Check sheet for the modelled part. Datum: model origin and axes. Units: mm. A direction names the side the tool comes from. Round coordinates to 2 decimals unless told otherwise and drop trailing zeros. Order: outer loops, then holes, each group sorted by start corner. A loop starts at its lowest first (then second) coordinate and runs counter-clockwise, first axis right, second up. Notation, with made-up numbers: M -17,41.25 L -2,41.25 A13 ccw -2,50.25 Z; hole C -36.5,-9.5 d7. An arc over 180 degrees is marked long. One line per item, written item: value. Start each with the question number.
(1) Cross-section at B-B, the plane y = 31. Enter the section's corners in (x, z), and give its area (3 significant figures).
(2) Cross-section at D-D, the plane z = 0. Enter the section's corners in (x, y).
(3) Cross-section at A-A, the plane z = 3.5. Enter the section's corners in (x, y).
(4) Access from +Z, -Z, +X, -X, +Y, -Y to the whole of each face (thin tool, end or side, straight path). Record for faces 5 (the face through (-8.4, 5.03, 7.11)), 6 (the face through (0, 0, 7)), 7 (the face through (15, 21.5, -8)), 8 (the face through (-0.225, 12.782, -9.635)), 9 (the face through (0, 21.5, 7)).
(5) Thickness scan on L1, parallel to X at y = 1.8, z = 0; L2, parallel to Z at x = -13.5, y = 1.8; L3, parallel to Z at x = -12, y = 6. Record the ranges inside material, lowest first.
(6) Depth check by flat-ended pin: pin 1 Ø1 at (x, z) = (2.5, 6.5) entering from +Y; pin 2 Ø5 at (y, z) = (9.5, 2) entering from +X; pin 3 Ø1.6 at (x, z) = (-2, -7) entering from +Y; pin 4 Ø0.7 at (x, y) = (-9, 22) entering from +Z. Enter the tip coordinate at first touch or a pass-through.
(7) Cross-section at C-C, the plane x = -13.5. Enter the section's corners in (y, z), and give its area (3 significant figures).
(8) Release check for a two-part mould opening along X. For faces 1 (the face through (-9.1, 21.4, -9.1)), 2 (the face through (-4.91, 7.606, -7.249)), 3 (the face through (-6.593, 22.291, -8.128)), 4 (the face through (-0.1, 10, -9.1)) record: released by +X, released by -X, zero draft, split by the parting line, or undercut.
from build123d import *

# Parameters (mm, degrees)
CROQUIS1_W                        = 5
CROQUIS1_H                        = 16.2
SALIENTE_EXTRUIR1_DEPTH           = 3
SALIENTE_EXTRUIR1_2_DEPTH         = 3
CROQUIS2_R                        = 0.8
CORTAR_EXTRUIR2_DEPTH             = 3
CROQUIS4_W                        = 32.2
CROQUIS4_H                        = 2
SALIENTE_EXTRUIR2_DEPTH           = 18.5
SALIENTE_EXTRUIR2_DEPTH_BACK      = 3
CROQUIS5_W                        = 5
CROQUIS5_H                        = 12.2
SALIENTE_EXTRUIR3_DEPTH           = 2
SALIENTE_EXTRUIR4_DEPTH           = 32.2
CORTAR_EXTRUIR3_REACH             = 35.7
CROQUIS8_W                        = 22.2
CROQUIS8_H                        = 2
CORTAR_EXTRUIR3_DIRECTION_2_DEPTH = 1
CORTAR_EXTRUIR4_REACH             = 20.2
CROQUIS9_R                        = 0.8
CROQUIS10_R                       = 0.8
SALIENTE_EXTRUIR5_DEPTH           = 2
SALIENTE_EXTRUIR7_DEPTH           = 32.2
CORTAR_EXTRUIR5_DEPTH             = 19.2
CORTAR_EXTRUIR9_DEPTH             = 0.3
CORTAR_EXTRUIR9_DIRECTION_2_REACH = 14.2
CROQUIS21_W                       = 32.2
CROQUIS21_H                       = 12.2
CORTAR_EXTRUIR10_DEPTH            = 0.4


with BuildPart() as part:
    # Croquis1 → Saliente-Extruir1 (new body)
    with BuildSketch(Plane(origin=(0, 0, 0), x_dir=(1, 0, 0), z_dir=(0, 1, 0))):
        with Locations((-13.6, 0)):
            Rectangle(CROQUIS1_W, CROQUIS1_H)
    extrude(amount=SALIENTE_EXTRUIR1_DEPTH)


with BuildPart() as body_2:
    # Croquis1 → Saliente-Extruir1 2 (new body)
    with BuildSketch(Plane(origin=(0, 0, 0), x_dir=(1, 0, 0), z_dir=(0, 1, 0))):
        with Locations((13.6, 0)):
            Rectangle(CROQUIS1_W, CROQUIS1_H)
    extrude(amount=SALIENTE_EXTRUIR1_2_DEPTH)


with BuildPart() as cortar_extruir2_tool:
    # Croquis2 → Cortar-Extruir2 (new body)
    with BuildSketch(Plane(origin=(0, 3, 0), x_dir=(1, 0, 0), z_dir=(0, 1, 0))):
        with Locations((-13.5, 0)):
            Circle(CROQUIS2_R)
        with Locations((14, 0)):
            Circle(CROQUIS2_R)
    extrude(amount=-CORTAR_EXTRUIR2_DEPTH)


with BuildPart() as part_1:
    add(part.part)

    # Cortar-Extruir2: cut by cortar_extruir2_tool
    add(cortar_extruir2_tool.part, mode=Mode.SUBTRACT)



with BuildPart() as body_2_1:
    add(body_2.part)

    # Cortar-Extruir2: cut by cortar_extruir2_tool
    add(cortar_extruir2_tool.part, mode=Mode.SUBTRACT)


with BuildPart() as part_2:
    add(part_1.part)

    add(body_2_1.part)  # Saliente-Extruir2 merges body 2
    # Croquis4 → Saliente-Extruir2 (add, two sides)
    with BuildSketch(Plane(origin=(0, 3, 0), x_dir=(1, 0, 0), z_dir=(0, 1, 0))) as saliente_extruir2_sk:
        with Locations((0, 7.1)):
            Rectangle(CROQUIS4_W, CROQUIS4_H)
        with Locations((0, -7.1)):
            Rectangle(CROQUIS4_W, CROQUIS4_H)
    extrude(amount=SALIENTE_EXTRUIR2_DEPTH)
    extrude(saliente_extruir2_sk.sketch, amount=-SALIENTE_EXTRUIR2_DEPTH_BACK)

    # Croquis5 → Saliente-Extruir3 (add)
    with BuildSketch(Plane.XY.offset(8.1)):
        with Locations((13.6, 27.6)):
            Rectangle(CROQUIS5_W, CROQUIS5_H)
        with Locations((-13.6, 27.6)):
            Rectangle(CROQUIS5_W, CROQUIS5_H)
    extrude(amount=-SALIENTE_EXTRUIR3_DEPTH)

    # Croquis7 → Saliente-Extruir4 (add, through all)
    with BuildSketch(Plane.ZY.offset(16.1)):
        with BuildLine():
            Line((10.1, 33.7), (8.1, 33.7))
            Line((8.1, 33.7), (8.1, 7.353005636))
            ThreePointArc((8.1, 7.353005636), (8.248733131, 9.983124325), (8.693036056, 12.579706844))
            Line((8.693036056, 12.579706844), (9.506963944, 16.120293156))
            ThreePointArc((9.506963944, 16.120293156), (9.951266869, 18.716875675), (10.1, 21.346994364))
            Line((10.1, 21.346994364), (10.1, 33.7))
        make_face()
    extrude(amount=-SALIENTE_EXTRUIR4_DEPTH)

    # Croquis8 → Cortar-Extruir3 (cut, up to next)
    with BuildSketch(Plane(origin=(0, 33.7, 0), x_dir=(1, 0, 0), z_dir=(0, 1, 0)), mode=Mode.PRIVATE) as cortar_extruir3_sk1:
        with Locations((0, -9.1)):
            Rectangle(CROQUIS8_W, CROQUIS8_H)
    cortar_extruir3_tool1 = extrude(cortar_extruir3_sk1.sketch, amount=-CORTAR_EXTRUIR3_REACH, mode=Mode.PRIVATE) & part_2.part
    add(cortar_extruir3_tool1.solids().sort_by_distance((0, 33.7, 9.1))[0], mode=Mode.SUBTRACT)

    # Croquis8 → Cortar-Extruir3 direction 2 (cut)
    with BuildSketch(Plane(origin=(0, 33.7, 0), x_dir=(1, 0, 0), z_dir=(0, 1, 0))):
        with Locations((0, -9.1)):
            Rectangle(CROQUIS8_W, CROQUIS8_H)
    extrude(amount=CORTAR_EXTRUIR3_DIRECTION_2_DEPTH, mode=Mode.SUBTRACT)

    # Croquis9 → Cortar-Extruir4 (cut, up to next)
    with BuildSketch(Plane.XY.offset(10.1), mode=Mode.PRIVATE) as cortar_extruir4_sk1:
        with Locations((-13.85, 27.95)):
            Circle(CROQUIS9_R)
    cortar_extruir4_tool1 = extrude(cortar_extruir4_sk1.sketch, amount=-CORTAR_EXTRUIR4_REACH, mode=Mode.PRIVATE) & part_2.part
    add(cortar_extruir4_tool1.solids().sort_by_distance((-13.85, 27.95, 10.1))[0], mode=Mode.SUBTRACT)
    # Croquis9 → Cortar-Extruir4 (cut, up to next)
    with BuildSketch(Plane.XY.offset(10.1), mode=Mode.PRIVATE) as cortar_extruir4_sk2:
        with Locations((13.85, 27.95)):
            Circle(CROQUIS9_R)
    cortar_extruir4_tool2 = extrude(cortar_extruir4_sk2.sketch, amount=-CORTAR_EXTRUIR4_REACH, mode=Mode.PRIVATE) & part_2.part
    add(cortar_extruir4_tool2.solids().sort_by_distance((13.85, 27.95, 10.1))[0], mode=Mode.SUBTRACT)

    # Croquis10 → Saliente-Extruir5 (add, symmetric)
    with BuildSketch(Plane(origin=(0, 0, -8.1), x_dir=(-1, 0, 0), z_dir=(0, 0, -1))):
        with BuildLine():
            Line((-10.633991508, 23.582443769), (-7.130262645, 28.458778116))
            ThreePointArc((-7.130262645, 28.458778116), (-5.478846803, 29.471128305), (-3.6, 29))
            Line((-3.6, 29), (2.4, 24.5))
            ThreePointArc((2.4, 24.5), (6.65658351, 22.269750529), (11.4, 21.5))
            Line((11.4, 21.5), (-14.694516799, 21.5))
            ThreePointArc((-14.694516799, 21.5), (-12.412826763, 22.050967456), (-10.633991508, 23.582443769))
        make_face()
        with Locations((-5.1, 27)):
            Circle(CROQUIS10_R, mode=Mode.SUBTRACT)
    extrude(amount=SALIENTE_EXTRUIR5_DEPTH, both=True)

    # Croquis13 → Saliente-Extruir7 (add, through all)
    with BuildSketch(Plane.ZY.offset(16.1)):
        with BuildLine():
            Line((-8.1, 21.5), (-10.1, 21.5))
            Line((-10.1, 21.5), (-10.1, 18.465682976))
            ThreePointArc((-10.1, 18.465682976), (-9.929666433, 15.016866347), (-9.420323649, 11.601618246))
            Line((-9.420323649, 11.601618246), (-8.779676351, 8.398381754))
            ThreePointArc((-8.779676351, 8.398381754), (-8.270333567, 4.983133653), (-8.1, 1.534317024))
            Line((-8.1, 1.534317024), (-8.1, 21.5))
        make_face()
    extrude(amount=-SALIENTE_EXTRUIR7_DEPTH)

    # Croquis14 → Cortar-Extruir5 (cut, through all)
    with BuildSketch(Plane.XY.offset(8.1)):
        with BuildLine():
            Line((-9, 15.116941663), (-9, 5.945455337))
            ThreePointArc((-9, 5.945455337), (-8.38417979, 5.022197037), (-7.295188221, 5.236060978))
            Line((-7.295188221, 5.236060978), (-2.457737974, 10.042262026))
            ThreePointArc((-2.457737974, 10.042262026), (-2.499999997, 10.499882305), (-2.457781062, 10.95750656))
            Line((-2.457781062, 10.95750656), (-7.290605641, 15.821753441))
            ThreePointArc((-7.290605641, 15.821753441), (-8.381186071, 16.041440002), (-9, 15.116941663))
        make_face()
        with BuildLine():
            Line((-5.263939022, 17.795188221), (-0.457737974, 12.957737974))
            ThreePointArc((-0.457737974, 12.957737974), (-0.000117695, 12.999999997), (0.45750656, 12.957781062))
            Line((0.45750656, 12.957781062), (5.321753441, 17.790605641))
            ThreePointArc((5.321753441, 17.790605641), (5.541440002, 18.881186071), (4.616941663, 19.5))
            Line((4.616941663, 19.5), (-4.554544663, 19.5))
            ThreePointArc((-4.554544663, 19.5), (-5.477802963, 18.88417979), (-5.263939022, 17.795188221))
        make_face()
        with BuildLine():
            Line((7.295188221, 15.763939022), (2.457737974, 10.957737974))
            ThreePointArc((2.457737974, 10.957737974), (2.499999997, 10.500117695), (2.457781062, 10.04249344))
            Line((2.457781062, 10.04249344), (7.290605641, 5.178246559))
            ThreePointArc((7.290605641, 5.178246559), (8.381186071, 4.958559998), (9, 5.883058337))
            Line((9, 5.883058337), (9, 15.054544663))
            ThreePointArc((9, 15.054544663), (8.38417979, 15.977802963), (7.295188221, 15.763939022))
        make_face()
        with BuildLine():
            Line((5.263939022, 3.204811779), (0.457737974, 8.042262026))
            ThreePointArc((0.457737974, 8.042262026), (0.000117695, 8.000000003), (-0.45750656, 8.042218938))
            Line((-0.45750656, 8.042218938), (-5.321753441, 3.209394359))
            ThreePointArc((-5.321753441, 3.209394359), (-5.541440002, 2.118813929), (-4.616941663, 1.5))
            Line((-4.616941663, 1.5), (4.554544663, 1.5))
            ThreePointArc((4.554544663, 1.5), (5.477802963, 2.11582021), (5.263939022, 3.204811779))
        make_face()
    extrude(amount=-CORTAR_EXTRUIR5_DEPTH, mode=Mode.SUBTRACT)

    # Croquis20 → Cortar-Extruir9 (cut)
    with BuildSketch(Plane(origin=(0, 21.5, 0), x_dir=(1, 0, 0), z_dir=(0, 1, 0))):
        Polygon((-12.4, 6.4), (-7.4, 6.4), (-7.4, 8.1), (-8.1, 8.1), (-8.1, 7.1), (-12.4, 7.1), align=None)
        Polygon((-7.4, 9.1), (-7.4, 9.8), (-12.4, 9.8), (-12.4, 8.1), (-11.7, 8.1), (-11.7, 9.1), align=None)
    extrude(amount=-CORTAR_EXTRUIR9_DEPTH, mode=Mode.SUBTRACT)

    # Croquis20 → Cortar-Extruir9 direction 2 (cut, up to next)
    with BuildSketch(Plane(origin=(0, 21.5, 0), x_dir=(1, 0, 0), z_dir=(0, 1, 0)), mode=Mode.PRIVATE) as cortar_extruir9_direction_2_sk1:
        Polygon((-12.4, 6.4), (-7.4, 6.4), (-7.4, 8.1), (-8.1, 8.1), (-8.1, 7.1), (-12.4, 7.1), align=None)
    cortar_extruir9_direction_2_tool1 = extrude(cortar_extruir9_direction_2_sk1.sketch, amount=CORTAR_EXTRUIR9_DIRECTION_2_REACH, mode=Mode.PRIVATE) & part_2.part
    add(cortar_extruir9_direction_2_tool1.solids().sort_by_distance((-9.541667, 21.5, -6.891667))[0], mode=Mode.SUBTRACT)
    # Croquis20 → Cortar-Extruir9 direction 2 (cut, up to next)
    with BuildSketch(Plane(origin=(0, 21.5, 0), x_dir=(1, 0, 0), z_dir=(0, 1, 0)), mode=Mode.PRIVATE) as cortar_extruir9_direction_2_sk2:
        Polygon((-7.4, 9.1), (-7.4, 9.8), (-12.4, 9.8), (-12.4, 8.1), (-11.7, 8.1), (-11.7, 9.1), align=None)
    cortar_extruir9_direction_2_tool2 = extrude(cortar_extruir9_direction_2_sk2.sketch, amount=CORTAR_EXTRUIR9_DIRECTION_2_REACH, mode=Mode.PRIVATE) & part_2.part
    add(cortar_extruir9_direction_2_tool2.solids().sort_by_distance((-10.258333, 21.5, -9.308333))[0], mode=Mode.SUBTRACT)

    # Croquis21 → Cortar-Extruir10 (cut)
    with BuildSketch(Plane(origin=(0, 3, 0), x_dir=(1, 0, 0), z_dir=(0, 1, 0))):
        Rectangle(CROQUIS21_W, CROQUIS21_H)
    extrude(amount=-CORTAR_EXTRUIR10_DEPTH, mode=Mode.SUBTRACT)


solid = part_2.part
Values found:
1. outline: M -16.1,6.1 L -11.1,6.1 L -11.1,10.1 L -16.1,10.1 Z; M 11.1,6.1 L 16.1,6.1 L 16.1,10.1 L 11.1,10.1 Z
1. area: 40.0 mm^2
2. outline: M -16.1,0 L -14.3,0 L -14.3,2.6 L -16.1,2.6 Z; M -12.7,0 L -11.1,0 L -11.1,2.6 L -12.7,2.6 Z; M 11.1,0 L 13.2,0 L 13.2,2.6 L 11.1,2.6 Z; M 14.8,0 L 16.1,0 L 16.1,2.6 L 14.8,2.6 Z
3. outline: M -16.1,0 L -11.1,0 L -11.1,2.6 L -16.1,2.6 Z; M 11.1,0 L 16.1,0 L 16.1,2.6 L 11.1,2.6 Z
4. face 5: +Z, -Z
4. face 6: +Z, -Z, +X, -X, -Y
4. face 7: -Z, +X, +Y
4. face 8: -Z, +X, -X, -Y
4. face 9: +Z, +Y
5. L1: -16.1 to -14.3, -12.7 to -11.1, 11.1 to 13.2, 14.8 to 16.1
5. L2: -8.1 to -0.8, 0.8 to 8.1
5. L3: -8.39 to -6.1, 6.1 to 8.1
6. pin 1: y = 21.5
6. pin 2: through
6. pin 3: y = 25.4
6. pin 4: z = -6.1
7. outline: M 0,-8.1 L 1.53,-8.1 A35 cw 8.4,-8.78 L 11.6,-9.42 A35 ccw 18.47,-10.1 L 21.5,-10.1 L 21.5,-6.1 L 2.6,-6.1 L 2.6,-0.8 L 0,-0.8 Z; M 0,0.8 L 2.6,0.8 L 2.6,6.1 L 27.23,6.1 L 27.23,10.1 L 21.35,10.1 A23.33 ccw 16.12,9.51 L 12.58,8.69 A23.33 cw 7.35,8.1 L 0,8.1 Z; M 28.67,6.1 L 33.7,6.1 L 33.7,10.1 L 28.67,10.1 Z
7. area: 194 mm^2
8. face 1: undercut
8. face 2: undercut
8. face 3: released by -X
8. face 4: zero draft
